Autodesk Inventor part; units mm, degrees
ref_plane "YZ Plane" through (0, 0, 0) normal (1, 0, 0) x (0, 1, 0)
ref_plane "XZ Plane" through (0, 0, 0) normal (0, 1, 0) x (-1, 0, 0)
ref_plane "XY Plane" through (0, 0, 0) normal (0, 0, 1) x (1, 0, 0)
sketch "Esquisse1" plane through (0, 0, 0) normal (0, 1, 0) x (-1, 0, 0)
  line L0 (0, 0) -> (30, 0)
  line L1 (30, 0) -> (30, -23)
  line L2 (28, -25) -> (2, -25)
  line L3 (0, -23) -> (0, 0)
  circle A0 centre (15, -12.5) radius 8.25
  line L4 (30, -23) -> (28, -25)
  line L5 (2, -25) -> (0, -23)
  point P0 (0, 0)
  point P1 (30, -25)
  point P2 (0, -25)
  point P3 (11.5, 0)
  point P4 (30, -4)
  point P5 (21, 0)
  point P6 (0, -2)
  point P7 (2, 0)
  dimension "d0" = 25
  dimension "d1" = 30
  dimension "d2" = 16.5
  dimension "d3" = 15
  dimension "d11" = 2
  dimension "d12" = 2
  dimension "d13" = 2
  dimension "d14" = 2
  dimension "d47" = 12.5
extrude "Extrusion1" add sketch "Esquisse1" along normal blind 3.5
sketch "Esquisse2" plane through (0, 3.5, 0) normal (0, 1, 0) x (1, 0, 0)
  circle A0 centre (-15, 12.5) radius 8.25 construction
  circle A1 centre (-15, 12.5) radius 10.8894 construction
  line L0 (-22.7, 4.8) -> (-22.7, 20.2) construction
  line L1 (-22.7, 20.2) -> (-7.3, 20.2) construction
  line L2 (-7.3, 20.2) -> (-7.3, 4.8) construction
  line L3 (-7.3, 4.8) -> (-22.7, 4.8) construction
  point P0 (0, 0)
  dimension "d19" = 15.4
  dimension "d20" = 15.4
hole "Perçage1" at (-22.7, 3.5, -4.8) at (-22.7, 3.5, -20.2) at (-7.3, 3.5, -20.2) at (-7.3, 3.5, -4.8) direction (0, -1, 0) diameter 2.4 end through all counterbore diameter 4.4 counterbore depth 2
sketch "Esquisse3" plane through (-30, 0, 0) normal (0, 0, 1) x (1, 0, 0)
  line L0 (0, 3.5) -> (30, 3.5)
  line L1 (0, 3.5) -> (30, 3.5)
  line L2 (30, 3.5) -> (30, -26.5)
  line L3 (30, -26.5) -> (0, -26.5)
  line L4 (0, -26.5) -> (0, 3.5)
  point P0 (30, 0)
  point P1 (30, 3.5)
  dimension "d29" = 30
  dimension "d48" = 30
  dimension "d49" = 30
extrude "Extrusion2" add sketch "Esquisse3" along normal blind 5
sketch "Esquisse4" plane through (-30, 0, -23) normal (-1, 0, 0) x (0, 0, 1)
  line L0 (0, 3.5) -> (28, 3.5)
  line L1 (28, 3.5) -> (0, 3.5)
  line L2 (0, 3.5) -> (0, 0)
  line L3 (0, 0) -> (-2, 0)
  line L4 (26.5, -26.5) -> (0, 0)
  line L5 (28, 3.5) -> (28, -26.5)
  line L6 (28, -26.5) -> (26.5, -26.5)
  line L7 (28, 3.5) -> (38, 3.5)
  line L8 (38, 3.5) -> (38, -26.5)
  line L9 (38, -26.5) -> (21.647, -26.5)
  point P0 (23, 0)
  point P1 (24.5, -21)
  point P2 (0, 3.5)
  point P3 (21, -21)
  dimension "d50" = 30
  dimension "d51" = 30
  dimension "d52" = 10
extrude "Extrusion3" add sketch "Esquisse4" along normal blind 2
sketch "Esquisse5" plane through (-30, 0, 0) normal (0, 0, -1) x (-1, 0, 0)
  line L0 (-5, -5) -> (-25, -5) construction
  line L1 (-25, -5) -> (-25, -20) construction
  line L2 (-25, -20) -> (-5, -20) construction
  line L3 (-5, -20) -> (-5, -5) construction
  line L4 (-28, 0) -> (-2, 0) construction
  line L5 (0, 0) -> (0, -23) construction
  point P0 (-30, 0)
  point P1 (0, -21)
  dimension "d36" = 15
  dimension "d37" = 20
  dimension "d38" = 5
  dimension "d39" = 5
hole "Perçage2" at (-25, -5, 0) at (-25, -20, 0) at (-5, -20, 0) at (-5, -5, 0) direction (0, 0, 1) diameter 3.4 end through all counterbore diameter 6.5 counterbore depth 3
equation "\"d3\" = 0.5 * d1"
equation "\"d47\" = 0.5 * d0"
equation "\"d20\" = d19"
equation "\"d48\" = d49"
equation "\"d51\" = d50"
properties part number "support nema8"
Source: CAD feature listing. Evaluate the final solid. Frame: model axes, mm. A direction names the side the tool comes from. Give positions to 0.01 mm unless a question says otherwise; leave off trailing zeros. Write each loop counter-clockwise with the first axis right and the second up, starting at its lowest first coordinate (ties: lowest second). Pieces come first, ordered by that corner, then holes. Notation, with made-up numbers: M 9.25,-2 L 30.25,-2 A20 ccw 30.25,5 Z; hole C 31,-32.5 d7. An arc over 180 degrees is marked long. Return JSON: item names as keys, results as strings. Group by question number.
1) Pin query (flat end, axial travel): P1, Ø7, axis at x = -7.3, z = -4.8, coming from the -Y side; P2, Ø5.5, axis at x = -5, y = -5, coming from the +Z side; P3, Ø3, axis at x = -25, y = -5, coming from the +Z side; P4, Ø5, axis at x = -25, y = -20, coming from the -Z side. Return the tip coordinate at first contact, or that it passes through.
2) Set-up query: faces 1 (the face through (-30, -25, 1)), 2 (the face through (-15, -13, 0)), 3 (the face through (-15, -11, 5)), 4 (the face through (-5.961, 2.486, -21.946)). Return all of +Z, -Z, +X, -X, +Y, -Y with unobstructed straight access to the full face (end or side cutting, diameter ignored); none if empty.
3) Cut plane B-B, the plane x = -15. Output: boundary loops of the cut face in (y, z), plus the area to 3 significant figures.
4) Cut plane A-A, the plane z = -12.5. Output: boundary loops of the cut face in (x, y), plus the area to 4 significant figures.
5) Pull-direction query (Z, two-part tool) for faces 5 (the face through (-18.807, 1.726, -5.181)), 6 (the face through (-1, 2, -24)), 7 (the face through (-15, 0, -4)); classes: pulls with the +Z half, pulls with the -Z half, needs draft (parallel to the pull), parting line crosses it, or undercut.
6) Material intervals for line 1 along Y through (x, z) = (-5, 4.2); line 2 along X through (y, z) = (-20, 2.25); line 3 along Y through (x, z) = (-4, 2), sorted ascending. Write a range as [from, to].
7) Cut plane D-D, the plane z = 4.5. Output: boundary loops of the cut face in (x, y).
8) Cut plane C-C, the plane y = -20. Output: boundary loops of the cut face in (x, z), plus the area to 3 significant figures.
Recorded:
{
 "1": {"P1": "stops at y = 0", "P2": "stops at z = 5", "P3": "passes through", "P4": "stops at z = 3"},
 "2": {"face 1": "-Z, -X, -Y", "face 2": "-Z, +X, -Y", "face 3": "+Z, +X, +Y, -Y", "face 4": "+Y"},
 "3": {"outline": "M -26.5,0 L 0,0 L 0,-4.25 L 3.5,-4.25 L 3.5,5 L -26.5,5 Z; M 0,-25 L 3.5,-25 L 3.5,-20.75 L 0,-20.75 Z", "area": "180 mm²"},
 "4": {"outline": "M -32,-10.5 L -30,-10.5 L -30,0 L -23.25,0 L -23.25,3.5 L -32,3.5 Z; M -6.75,0 L 0,0 L 0,3.5 L -6.75,3.5 Z", "area": "75.25 mm²"},
 "5": {"face 5": "undercut", "face 6": "pulls with the -Z half", "face 7": "needs draft"},
 "6": {"line 1": "y = [-26.5, -21.7], [-18.3, -6.7], [-3.3, 3.5]", "line 2": "x = [-32, -28.25], [-21.75, -8.25], [-1.75, 0]", "line 3": "y = [-26.5, -23.09], [-16.91, -8.09], [-1.91, 3.5]"},
 "7": {"outline": "M -32,-26.5 L 0,-26.5 L 0,3.5 L -32,3.5 Z; hole C -25,-20 d3.4; hole C -25,-5 d3.4; hole C -5,-20 d3.4; hole C -5,-5 d3.4"},
 "8": {"outline": "M -32,-3 L -30,-3 L -30,0 L -28.25,0 L -28.25,3 L -26.7,3 L -26.7,5 L -30,5 L -30,15 L -32,15 Z; M -23.3,3 L -21.75,3 L -21.75,0 L -8.25,0 L -8.25,3 L -6.7,3 L -6.7,5 L -23.3,5 Z; M -3.3,3 L -1.75,3 L -1.75,0 L 0,0 L 0,5 L -3.3,5 Z", "area": "133 mm²"}
}
